Verification items for the finished model (mm, model axes). A direction names the side the tool comes from. Coordinates: 2 decimals unless noted, no trailing zeros. Order: outer loops, then holes, each group sorted by start corner. A loop starts at its lowest first (then second) coordinate and runs counter-clockwise, first axis right, second up. Notation, with made-up numbers: M -34,75.25 L 7,75.25 A8 ccw 7,83.25 Z; hole C 76.25,-37 d8. An arc over 180 degrees is marked long. Return JSON: item names as keys, results as strings. Group by question number.
Q1. Access from +Z, -Z, +X, -X, +Y, -Y to the whole of each face (thin tool, end or side, straight path). Record for faces 1 (the face through (-31.354, 0.676, 3.648)), 2 (the face through (-27.5, 12.2, 3.6)), 3 (the face through (28, -19.82, 4)), 4 (the face through (33.632, -12, 6)), 5 (the face through (36.232, 12, 4)).
Q2. Mould release check, pull along Z, two halves, no side actions. Record for faces 6 (the face through (22.19, -13.03, 8.32)), 7 (the face through (22.037, 13.01, 8.157)), 8 (the face through (-30, -5, 4)), 9 (the face through (34.95, 12.24, 6.52)): pulls with the +Z half, pulls with the -Z half, needs draft (parallel to the pull), parting line crosses it, or undercut.
Q3. Section check B-B, the plane x = 0. Enter the section's corners in (y, z).
Q4. Thickness scan on probe 1 along Y at (x, z) = (0, 5); probe 2 along Y at (x, z) = (0, 8.55); probe 3 along X at (y, z) = (-1.5, 6). Record the ranges inside material, lowest first.
Q5. Section check A-A, the plane z = 2.5. Enter the section's corners in (x, y).
Q6. Go/stop test with flat-tipped pins: pin 1 Ø4 at (y, z) = (9.5, 6.5) entering from +X; pin 2 Ø1 at (y, z) = (-14, 3.5) entering from -X; pin 3 Ø3.5 at (y, z) = (-11.93, 9.33) entering from -X. Record where each tip stops, or that it passes through.
Q7. Section check D-D, the plane y = 6. Enter the section's corners in (x, z).
Q8. Section check C-C, the plane y = 0. Enter the section's corners in (x, z), then the cut area to 3 significant figures.
from build123d import *

# Parameters (mm, degrees)
CROQUIS1_R                 = 2.25
SALIENTE_EXTRUIR1_DEPTH    = 7.4
CROQUIS4_R                 = 5.5
CORTAR_EXTRUIR2_DEPTH      = 3
CROQUIS5_R                 = 2.9
CORTAR_EXTRUIR3_DEPTH      = 4
CROQUIS2_R                 = 20.5
CORTAR_EXTRUIR1_DEPTH      = 49.036098674
CROQUIS3_R                 = 27.65
CROQUIS3_R_2               = 23
SALIENTE_EXTRUIR2_DEPTH    = 4.8
CORTAR_EXTRUIR4_DEPTH      = 20
CORTAR_EXTRUIR4_DEPTH_BACK = 9
CROQUIS6_R                 = 1.5


with BuildPart() as part:
    # Croquis1 → Saliente-Extruir1 (new body)
    with BuildSketch(Plane.XY):
        with BuildLine():
            Line((-35.955174002, 4.355699785), (-18.80791724, 20.267825466))
            ThreePointArc((-18.80791724, 20.267825466), (0.325119352, 27.648088495), (19.279317337, 19.819950126))
            Line((19.279317337, 19.819950126), (36.231616172, 19.819950126))
            Line((36.231616172, 19.819950126), (36.231616172, 4.279499518))
            ThreePointArc((36.231616172, 4.279499518), (38.576991534, 0), (36.231616172, -4.279499518))
            Line((36.231616172, -4.279499518), (36.231616172, -19.819950126))
            Line((36.231616172, -19.819950126), (19.279317337, -19.819950126))
            ThreePointArc((19.279317337, -19.819950126), (-8.400531281, -26.34299858), (-27.194162977, -5))
            Line((-27.194162977, -5), (-33.5, -5))
            ThreePointArc((-33.5, -5), (-38.336243321, -1.269153473), (-35.955174002, 4.355699785))
        make_face()
        with Locations((-33.5, 0)):
            Circle(CROQUIS1_R, mode=Mode.SUBTRACT)
        with Locations((33.5, 0)):
            Circle(CROQUIS1_R, mode=Mode.SUBTRACT)
    extrude(amount=SALIENTE_EXTRUIR1_DEPTH)

    # Croquis4 → Cortar-Extruir2 (cut)
    with BuildSketch(Plane(origin=(33.631616172, 0, 0), x_dir=(0, -0.9996578345310084, -0.026157481927263488), z_dir=(1, 0, 0))):
        with Locations((-12.445697835, -9.09891785)):
            Circle(CROQUIS4_R)
        with Locations((11.67759578, -9.64152027)):
            Circle(CROQUIS4_R)
    extrude(amount=-CORTAR_EXTRUIR2_DEPTH, mode=Mode.SUBTRACT)

    # Croquis5 → Cortar-Extruir3 (cut)
    with BuildSketch(Plane(origin=(36.231616172, 0, 0), x_dir=(0, -1, 0), z_dir=(-1, 0, 0))):
        with Locations((-12.203434568, 9.42135263)):
            Circle(CROQUIS5_R)
        with Locations((11.925798003, 9.332764774)):
            Circle(CROQUIS5_R)
    extrude(amount=CORTAR_EXTRUIR3_DEPTH, mode=Mode.SUBTRACT)

    # Croquis2 → Cortar-Extruir1 (cut, through all)
    with BuildSketch(Plane.XY.offset(7.4)):
        Circle(CROQUIS2_R)
    extrude(amount=-CORTAR_EXTRUIR1_DEPTH, mode=Mode.SUBTRACT)

    # Croquis3 → Saliente-Extruir2 (add)
    with BuildSketch(Plane.XY.offset(7.4)):
        with Locations(Location((0, 0, 0), (0, 0, 190.41821508))):
            Circle(CROQUIS3_R)
        Circle(CROQUIS3_R_2, mode=Mode.SUBTRACT)
    extrude(amount=SALIENTE_EXTRUIR2_DEPTH)

    # Croquis6 → Cortar-Extruir4 (cut, two sides: drawn at the far end of the back side and taken through both)
    with BuildSketch(Plane(origin=(26.031616172, 0, 0), x_dir=(0, -1, 0), z_dir=(-1, 0, 0)).offset(-CORTAR_EXTRUIR4_DEPTH_BACK)):
        with Locations(Location((-12.203434568, 9.42135263, 0), (0, 0, 180))):
            Circle(CROQUIS6_R)
        with Locations(Location((11.925798003, 9.332764774, 0), (0, 0, 180))):
            Circle(CROQUIS6_R)
    extrude(amount=CORTAR_EXTRUIR4_DEPTH + CORTAR_EXTRUIR4_DEPTH_BACK, mode=Mode.SUBTRACT)


solid = part.part
Numbers:
{
 "1": {"face 1": "+Z, -Z", "face 2": "+Z, -Z, -X, +Y", "face 3": "+Z, -Z, +X, -Y", "face 4": "+Z", "face 5": "+Z, -Z, +X, +Y"},
 "2": {"face 6": "undercut", "face 7": "undercut", "face 8": "needs draft", "face 9": "pulls with the +Z half"},
 "3": {"outline": "M -27.65,0 L -20.5,0 L -20.5,7.4 L -23,7.4 L -23,12.2 L -27.65,12.2 Z; M 20.5,0 L 27.65,0 L 27.65,12.2 L 23,12.2 L 23,7.4 L 20.5,7.4 Z"},
 "4": {"probe 1": "y = -27.65 to -20.5, 20.5 to 27.65", "probe 2": "y = -27.65 to -23, 23 to 27.65", "probe 3": "x = -38.27 to -35.18, -31.82 to -20.45, 20.45 to 31.82, 35.18 to 38.35"},
 "5": {"outline": "M -35.96,4.36 A5 ccw -33.5,-5 L -27.19,-5 A27.65 ccw 19.28,-19.82 L 36.23,-19.82 L 36.23,-4.28 A5.08 ccw 36.23,4.28 L 36.23,19.82 L 19.28,19.82 A27.65 ccw -18.81,20.27 Z; hole C -33.5,0 d4.5; hole C 0,0 d41; hole C 33.5,0 d4.5"},
 "6": {"pin 1": "stops at x = 36.23", "pin 2": "stops at x = -24.13", "pin 3": "stops at x = -25.71"},
 "7": {"outline": "M -34.18,0 L -19.6,0 L -19.6,7.4 L -22.2,7.4 L -22.2,12.2 L -26.99,12.2 L -26.99,7.4 L -34.18,7.4 Z; M 19.6,0 L 36.23,0 L 36.23,7.4 L 26.99,7.4 L 26.99,12.2 L 22.2,12.2 L 22.2,7.4 L 19.6,7.4 Z"},
 "8": {"outline": "M -38.5,0 L -35.75,0 L -35.75,7.4 L -38.5,7.4 Z; M -31.25,0 L -20.5,0 L -20.5,7.4 L -23,7.4 L -23,12.2 L -27.65,12.2 L -27.65,7.4 L -31.25,7.4 Z; M 20.5,0 L 31.25,0 L 31.25,7.4 L 27.65,7.4 L 27.65,12.2 L 23,12.2 L 23,7.4 L 20.5,7.4 Z; M 35.75,0 L 38.58,0 L 38.58,7.4 L 35.75,7.4 Z", "area": "245 mm2"}
}
